```python
from build123d import *

# Parameters (mm, degrees)
SKETCH1_W           = 25
SKETCH1_H           = 16.5
SKETCH1_R           = 1.1
BOSS_EXTRUDE3_DEPTH = 3.175
SKETCH4_W           = 14.012619733
SKETCH4_H           = 3.256845332
BOSS_EXTRUDE4_DEPTH = 7.62
RIB13_REACH         = 22.577
SKETCH8_WALL_W      = 52.139653992
SKETCH8_WALL_H      = 2.54
SKETCH11_R          = 1.1
CUT_EXTRUDE3_DEPTH  = 22.341270784


with BuildPart() as part:
    # Sketch1 → Boss-Extrude3 (new body)
    with BuildSketch(Plane.XY):
        with Locations((0.288145608, 3.722304951)):
            Rectangle(SKETCH1_W, SKETCH1_H)
        with Locations((-10.211854392, 9.972304951)):
            Circle(SKETCH1_R, mode=Mode.SUBTRACT)
        with Locations((-10.211854392, -2.527695049)):
            Circle(SKETCH1_R, mode=Mode.SUBTRACT)
        with Locations((10.788145608, 9.972304951)):
            Circle(SKETCH1_R, mode=Mode.SUBTRACT)
        with Locations((10.788145608, -2.527695049)):
            Circle(SKETCH1_R, mode=Mode.SUBTRACT)
    extrude(amount=-BOSS_EXTRUDE3_DEPTH)

    # Sketch4 → Boss-Extrude4 (add)
    with BuildSketch(Plane(origin=(0, 0, -3.175), x_dir=(-1, 0, 0), z_dir=(0, 0, -1))):
        with Locations((-0.142456745, -2.899272383)):
            Rectangle(SKETCH4_W, SKETCH4_H)
    extrude(amount=BOSS_EXTRUDE4_DEPTH)

    # Sketch8 wall → Rib13 (add, up to next)
    with BuildSketch(Plane(origin=(0, 2.497441859, -5.961770268), x_dir=(0, -0.784409210178, -0.620243654533), z_dir=(0, 0.620243654533, -0.784409210178)), mode=Mode.PRIVATE) as rib13_sk1:
        Rectangle(SKETCH8_WALL_W, SKETCH8_WALL_H)
    rib13_tool1 = extrude(rib13_sk1.sketch, amount=-RIB13_REACH, mode=Mode.PRIVATE) - part.part
    add(rib13_tool1.solids().sort_by_distance((0, 2.497441859, -5.961770268))[0])

    # Sketch11 → Cut-Extrude3 (cut, through all)
    with BuildSketch(Plane(origin=(0, -1.270849717, 0), x_dir=(1, 0, 0), z_dir=(0, 1, 0))):
        with Locations(Location((-4.863853122, 8.795, 0), (0, 0, 270))):
            Circle(SKETCH11_R)
        with Locations(Location((5.148766611, 8.795, 0), (0, 0, 270))):
            Circle(SKETCH11_R)
    extrude(amount=-CUT_EXTRUDE3_DEPTH, mode=Mode.SUBTRACT)


solid = part.part
```
Source: CAD feature listing. Evaluate the final solid. Frame: model axes, mm. A direction names the side the tool comes from. Coordinates: 2 decimals unless noted, no trailing zeros. Write each loop counter-clockwise with the first axis right and the second up, starting at its lowest first coordinate (ties: lowest second). Pieces come first, ordered by that corner, then holes. Notation, with made-up numbers: (7, 41) -> (14, 41) arc R13 ccw to (14, 47) -> close; hole circle Ø2 at (45, 58). An arc over 180 degrees is marked (long way). Return JSON: item names as keys, results as strings. Group by question number.
1) Section query C-C, the plane x = -10. Return loops of the section in (y, z) (3 decimals).
2) Section query D-D, the plane z = -6.5. Return loops of the section in (x, y), plus the area to 3 significant figures.
3) Section query A-A, the plane y = -2. Return loops of the section in (x, z) (3 decimals), plus the area to 3 significant figures.
4) Set-up query: faces 5 (the face through (2, -1.271, -7)), 6 (the face through (1.27, 1, -5)), 7 (the face through (7.149, -3, -7)), 8 (the face through (-1.27, 1, -5)), 9 (the face through (-6.864, -3, -7)). Return all of +Z, -Z, +X, -X, +Y, -Y with unobstructed straight access to the full face (end or side cutting, diameter ignored); none if empty.
5) Ray query, line 1 along Y through (x, z) = (-9.5, -2.75); line 2 along X through (y, z) = (3.25, -4); line 3 along Z through (x, y) = (-9, 9.5) (3 decimals). Return the intervals inside material, ascending.
6) Contact query for flat-ended pins moving along their axis: P1, Ø3, axis at y = 2, z = -6.5, coming from the -X side; P2, Ø1.5, axis at x = -2.5, y = 9.5, coming from the -Z side (3 decimals); P3, Ø1.3, axis at x = -10.21, y = 9.97, coming from the -Z side; P4, Ø2.5, axis at y = -2.5, z = -6.5, coming from the -X side. Output: stop coordinate, or through.
7) Section query B-B, the plane x = 4.75. Return loops of the section in (y, z) (3 decimals).
8) Mould query, pull axis X, two halves, no side actions, for faces 1 (the face through (-12.212, 4, -2)), 2 (the face through (0, 4, 0)), 3 (the face through (9.69, -2.48, -1.57)), 4 (the face through (9.98, 10.72, -1.57)). Classes: +X half, -X half, draft (parallel to the pull), parting line (faces both ways), or undercut.
From the geometry:
{
 "1": {"outline": "(-4.528, -3.175) -> (-3.607, -3.175) -> (-3.607, 0) -> (-4.528, 0) -> close; (-1.448, -3.175) -> (8.893, -3.175) -> (8.893, 0) -> (-1.448, 0) -> close; (11.052, -3.175) -> (11.972, -3.175) -> (11.972, 0) -> (11.052, 0) -> close"},
 "2": {"outline": "(-6.86, -4.53) -> (7.15, -4.53) -> (7.15, -1.27) -> (1.27, -1.27) -> (1.27, 1.82) -> (-1.27, 1.82) -> (-1.27, -1.27) -> (-6.86, -1.27) -> close", "area": "53.5 mm²"},
 "3": {"outline": "(-12.212, -3.175) -> (-11.177, -3.175) -> (-11.177, 0) -> (-12.212, 0) -> close; (-9.247, -3.175) -> (-6.864, -3.175) -> (-6.864, -10.795) -> (7.149, -10.795) -> (7.149, -3.175) -> (9.823, -3.175) -> (9.823, 0) -> (-9.247, 0) -> close; (11.753, -3.175) -> (12.788, -3.175) -> (12.788, 0) -> (11.753, 0) -> close; hole circle Ø2.2 at (-4.864, -8.795); hole circle Ø2.2 at (5.149, -8.795)", "area": "166 mm²"},
 "4": {"face 5": "-Z, +Y", "face 6": "-Z, +X, +Y", "face 7": "-Z, +X, +Y, -Y", "face 8": "-Z, -X, +Y", "face 9": "-Z, -X, +Y, -Y"},
 "5": {"line 1": "-4.53 to -3.37, -1.69 to 9.13, 10.81 to 11.97", "line 2": "-1.27 to 1.27", "line 3": "-3.175 to 0"},
 "6": {"P1": "x = -1.27", "P2": "z = -3.175", "P3": "through", "P4": "x = -6.86"},
 "7": {"outline": "(-4.528, -10.795) -> (-1.271, -10.795) -> (-1.271, -9.82) -> (-4.528, -9.82) -> close; (-4.528, -7.77) -> (-1.271, -7.77) -> (-1.271, -3.175) -> (11.972, -3.175) -> (11.972, 0) -> (-4.528, 0) -> close"},
 "8": {"face 1": "-X half", "face 2": "draft", "face 3": "undercut", "face 4": "undercut"}
}
